from build123d import *

# Parameters (mm, degrees)
SALIENTE_EXTRUIR2_DEPTH = 10


with BuildPart() as part:
    # Croquis1 → Saliente-Extruir2 (new body)
    with BuildSketch(Plane.XY):
        with BuildLine():
            ThreePointArc((-38.687161159, 0.254415054), (-39.39426794, 0.547308273), (-39.687161159, 1.254415054))
            Line((-39.687161159, 1.254415054), (-39.687161159, 24.254415054))
            ThreePointArc((-39.687161159, 24.254415054), (-39.39426794, 24.961521836), (-38.687161159, 25.254415054))
            Line((-38.687161159, 25.254415054), (-1.187161159, 25.254415054))
            Line((-1.187161159, 25.254415054), (-1.187161159, 28.254415054))
            Line((-1.187161159, 28.254415054), (-39.187161159, 28.254415054))
            ThreePointArc((-39.187161159, 28.254415054), (-42.015588284, 27.082842179), (-43.187161159, 24.254415054))
            Line((-43.187161159, 24.254415054), (-43.187161159, -3.245584946))
            Line((-43.187161159, -3.245584946), (-43.187161159, -4.245584946))
            ThreePointArc((-43.187161159, -4.245584946), (-44.358734034, -7.07401207), (-47.187161159, -8.245584946))
            Line((-47.187161159, -8.245584946), (-55.187161159, -8.245584946))
            Line((-55.187161159, -8.245584946), (-55.187161159, -11.745584946))
            Line((-55.187161159, -11.745584946), (-43.187161159, -11.745584946))
            Line((-43.187161159, -11.745584946), (-39.687161159, -11.745584946))
            Line((-39.687161159, -11.745584946), (-39.687161159, -5.245584946))
            ThreePointArc((-39.687161159, -5.245584946), (-39.101374721, -3.831371383), (-37.687161159, -3.245584946))
            Line((-37.687161159, -3.245584946), (-1.187161159, -3.245584946))
            Line((-1.187161159, -3.245584946), (-1.187161159, 0.254415054))
            Line((-1.187161159, 0.254415054), (-38.687161159, 0.254415054))
        make_face()
    saliente_extruir2 = extrude(amount=SALIENTE_EXTRUIR2_DEPTH)

    # Simetría2: Saliente-Extruir2 across plane
    add(saliente_extruir2.mirror(Plane(origin=(-1.187161159, 0, 10), x_dir=(0, 0, 1), z_dir=(-1, 0, 0))))


solid = part.part
Build history of the part. All positions in model axes, mm. A direction names the side the tool comes from. Give positions to 0.01 mm unless a question says otherwise; leave off trailing zeros. Order: outer loops, then holes, each group sorted by start corner. A loop starts at its lowest first (then second) coordinate and runs counter-clockwise, first axis right, second up. Notation, with made-up numbers: M 86,88.5 L 92,88.5 A12 ccw 92,105.5 Z; hole C -20.5,28.5 d5. An arc over 180 degrees is marked long. Put each result on its own line as item: value.
Item 1: Slice it at A-A, the plane y = 12. Write the cut outline in (x, z), plus the area to 3 significant figures.
From the geometry:
outline: M -43.19,0 L -39.69,0 L -39.69,10 L -43.19,10 Z; M 37.31,0 L 40.81,0 L 40.81,10 L 37.31,10 Z
area: 70.0 mm2
Item 2: Flat gauge pins, fed straight in: pin 1 Ø4 at (y, z) = (1.5, 1.5) entering from +X; pin 2 Ø2 at (y, z) = (8, 5.5) entering from -X; pin 3 Ø3 at (x, z) = (11.5, 6.5) entering from -Y. Where does each tip first touch, or does it go through?
From the geometry:
pin 1: stops at x = 40.81
pin 2: stops at x = -43.19
pin 3: stops at y = -3.25
Item 3: Slice it at C-C, the plane x = -14. Write the cut outline in (y, z).
From the geometry:
outline: M -3.25,0 L 0.25,0 L 0.25,10 L -3.25,10 Z; M 25.25,0 L 28.25,0 L 28.25,10 L 25.25,10 Z
Item 4: Slice it at D-D, the plane y = -1. Write the cut outline in (x, z).
From the geometry:
outline: M -43.19,0 L 40.81,0 L 40.81,10 L -43.19,10 Z
Item 5: 3-axis set-ups, long thin cutter, end or side, ignore diameter. For faces 1 (the flat face through (37.313, -9, 5)), 2 (the flat face through (49, -8.246, 5)), 3 (the flat face through (-43.187, 10, 5)): which of +Z, -Z, +X, -X, +Y, -Y reach the whole face in a straight line?
From the geometry:
face 1: +Z, -Z, -Y
face 2: +Z, -Z, +X, +Y
face 3: +Z, -Z, -X, +Y
Item 6: Slice it at B-B, the plane z = 3. Write the cut outline in (x, y), plus the area to 3 significant figures.
From the geometry:
outline: M -55.19,-11.75 L -39.69,-11.75 L -39.69,-5.25 A2 cw -37.69,-3.25 L 35.31,-3.25 A2 cw 37.31,-5.25 L 37.31,-11.75 L 52.81,-11.75 L 52.81,-8.25 L 44.81,-8.25 A4 cw 40.81,-4.25 L 40.81,24.25 A4 ccw 36.81,28.25 L -39.19,28.25 A4 ccw -43.19,24.25 L -43.19,-4.25 A4 cw -47.19,-8.25 L -55.19,-8.25 Z; hole M -39.69,1.25 A1 ccw -38.69,0.25 L 36.31,0.25 A1 ccw 37.31,1.25 L 37.31,24.25 A1 ccw 36.31,25.25 L -38.69,25.25 A1 ccw -39.69,24.25 Z
area: 867 mm2
Item 7: Two-plate mould, pull along Y, no slides. Class faces 4 (the cylindrical face through (-39.12, -3.85, 4.93)), 5 (the flat face through (40.813, 10, 5)), 6 (the flat face through (-2, 0.254, 5)): +Y half, -Y half, draft (parallel to the pull), parting line (faces both ways), or undercut.
From the geometry:
face 4: -Y half
face 5: draft
face 6: undercut
Item 8: Probe line 1 (Y direction, x = -30.5, z = 7.5); line 2 (X direction, y = 21, z = 2); line 3 (Y direction, x = 36.5, z = 9). List the from-to ranges inside material, lowest first. Write a range as [from, to].
From the geometry:
line 1: y = [-3.25, 0.25], [25.25, 28.25]
line 2: x = [-43.19, -39.69], [37.31, 40.81]
line 3: y = [-3.64, 0.27], [25.24, 28.25]
